Could you check a few things on this model? Use its own coordinates, in mm. Face numbers are marked on the shaded views. A direction names the side the tool comes from. Round coordinates to 2 decimals unless told otherwise and drop trailing zeros. Write each loop counter-clockwise with the first axis right and the second up, starting at its lowest first coordinate (ties: lowest second). Pieces come first, ordered by that corner, then holes. Notation, with made-up numbers: (-2, -14) -> (17, -14) arc R21 cw to (17, 14) -> close; hole circle Ø1 at (-33, -15). An arc over 180 degrees is marked (long way). Answer in a Markdown table with one row per item. Add a question column.
```python
from build123d import *

# Parameters (mm, degrees)
EXTRUDE_1_DEPTH     = 7
SKETCH_2_R          = 10.375
CUT_EXTRUDE_1_DEPTH = 3.5
SKETCH_6_R          = 5
CUT_EXTRUDE_2_DEPTH = 48.095647357
EXTRUDE_START       = 6.2
SKETCH_8_R          = 5
EXTRUDE_2_DEPTH     = 6.2


with BuildPart() as part:
    # 草图1 → 凸台-拉伸1 (new body)
    with BuildSketch(Plane.XY):
        with BuildLine():
            Line((2.1, 11.814821201), (40.875, 4.922842167))
            ThreePointArc((40.875, 4.922842167), (45, 0), (40.875, -4.922842167))
            Line((40.875, -4.922842167), (2.1, -11.814821201))
            ThreePointArc((2.1, -11.814821201), (-12, 0), (2.1, 11.814821201))
        make_face()
    extrude(amount=EXTRUDE_1_DEPTH)

    # 草图2 → 切除-拉伸1 (cut)
    with BuildSketch(Plane.XY.offset(7)):
        Circle(SKETCH_2_R)
    extrude(amount=-CUT_EXTRUDE_1_DEPTH, mode=Mode.SUBTRACT)

    # 草图6 → 切除-拉伸2 (cut, through all)
    with BuildSketch(Plane(origin=(0, 0, 0), x_dir=(-1, 0, 0), z_dir=(0, 0, -1))):
        Circle(SKETCH_6_R)
    extrude(amount=-CUT_EXTRUDE_2_DEPTH, mode=Mode.SUBTRACT)

    # 草图8 → 凸台-拉伸2 (add)
    with BuildSketch(Plane(origin=(0, 0, 0), x_dir=(-1, 0, 0), z_dir=(0, 0, -1)).offset(EXTRUDE_START)):
        with Locations((-40, 0)):
            Circle(SKETCH_8_R)
    extrude(amount=-EXTRUDE_2_DEPTH)

    # 草图9 → 切除-旋转1 (revolve, cut)
    with BuildSketch(Plane(origin=(0, 0, 0), x_dir=(1, 0, 0), z_dir=(0, 1, 0))):
        Polygon((40, 6.2), (38, 6.2), (38, 2.7), (36, 2.7), (36, -7), (40, -7), align=None)
    revolve(axis=Axis((40, 0, -14.45), (0, 0, 1)), mode=Mode.SUBTRACT)


solid = part.part
```
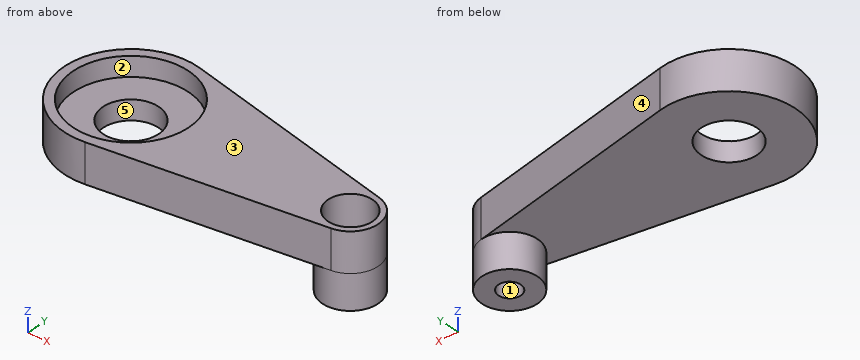
(1) For P1, Ø4, axis at x = 2, z = -1.5, coming from the -Y side; P2, Ø10.5, axis at x = 4, y = -2.5, coming from the +Z side; P3, Ø4, axis at x = 39, y = 0, coming from the +Z side; P4, Ø9, axis at x = 0, y = 0, coming from the -Z side, each with a flat end and sliding along its axis, tell me the tip position at first contact or that it passes through.
(2) Suppose I cut it at C-C, the plane z = 6.25. Please give me the cut outline in (x, y) (3 decimals).
(3) If we mould it in two halves opening along Y, with no side actions, what happens to the marked faces 3, 4 and 5? For each: pulls with the +Y half, pulls with the -Y half, needs draft (parallel to the pull), parting line crosses it, or undercut.
(4) Suppose I cut it at A-A, the plane x = 0. Please give me the cut outline in (y, z) (3 decimals), then the cut area to 3 significant figures.
(5) On a 3-axis mill with a long thin cutter (end or side, diameter ignored), from which of +Z, -Z, +X, -X, +Y, -Y can I reach the whole of each face in a straight line? I mean the marked faces 1 and 2. Say none if no direction works.
(6) I need wall thicknesses on L1, parallel to X at y = -3.5, z = 1.75; L2, parallel to Y at x = 40, z = -4.25; L3, parallel to Z at x = 10, y = 5.25. Which ranges of each line are inside material? Lowest first, please.
(7) Suppose I cut it at B-B, the plane y = 0. Please give me the cut outline in (x, z) (3 decimals).
(8) Suppose I cut it at D-D, the plane z = -4.75. Please give me the cut outline in (x, y), then the cut area to 3 significant figures.
Response:
| question | item | result |
|---|---|---|
| 1 | P1 | y = -11.98 |
| 1 | P2 | z = 3.5 |
| 1 | P3 | z = -2.7 |
| 1 | P4 | through |
| 2 | outline | (2.1, -11.815) -> (40.875, -4.923) arc R5 ccw to (40.875, 4.923) -> (2.1, 11.815) arc R12 ccw (long way) to start; hole circle Ø20.75 at (0, 0); hole circle Ø8 at (40, 0) |
| 3 | face 3 | needs draft |
| 3 | face 4 | pulls with the +Y half |
| 3 | face 5 | undercut |
| 4 | outline | (-12, 0) -> (-5, 0) -> (-5, 3.5) -> (-10.375, 3.5) -> (-10.375, 7) -> (-12, 7) -> close; (5, 0) -> (12, 0) -> (12, 7) -> (10.375, 7) -> (10.375, 3.5) -> (5, 3.5) -> close |
| 4 | area | 60.4 mm² |
| 5 | face 1 | +Z, -Z |
| 5 | face 2 | +Z |
| 6 | L1 | -11.48 to -3.57, 3.57 to 38.06, 41.94 to 43.57 |
| 6 | L2 | -5 to -2, 2 to 5 |
| 6 | L3 | 0 to 7 |
| 7 | outline | (-12, 0) -> (-5, 0) -> (-5, 3.5) -> (-10.375, 3.5) -> (-10.375, 7) -> (-12, 7) -> close; (5, 0) -> (35, 0) -> (35, -6.2) -> (38, -6.2) -> (38, -2.7) -> (36, -2.7) -> (36, 7) -> (10.375, 7) -> (10.375, 3.5) -> (5, 3.5) -> close; (42, -6.2) -> (45, -6.2) -> (45, 7) -> (44, 7) -> (44, -2.7) -> (42, -2.7) -> close |
| 8 | outline | circle Ø10 at (40, 0); hole circle Ø4 at (40, 0) |
| 8 | area | 66.0 mm² |
